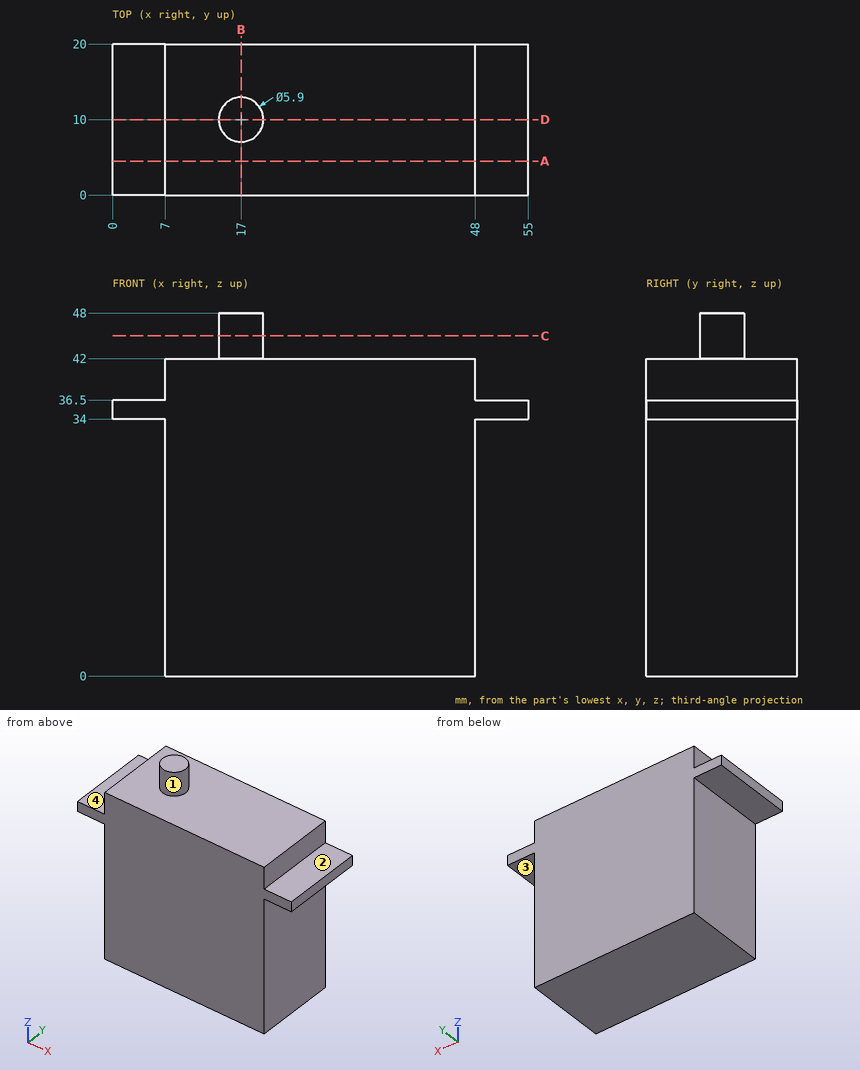
Here's the drawing with two shaded views (mm, measured from the low corner). I have some questions. A direction names the side the tool comes from. Give positions to 0.01 mm unless a question says otherwise; leave off trailing zeros. Order: outer loops, then holes, each group sorted by start corner. A loop starts at its lowest first (then second) coordinate and runs counter-clockwise, first axis right, second up. Notation, with made-up numbers: (72, 55) -> (79, 55) arc R35 cw to (79, 93) -> close; hole circle Ø6 at (89, -15.75). An arc over 180 degrees is marked (long way). One line per item, written item: value. Start each with the question number.
1. Will these pins go through, and if not, where does the flat tip stop? pin 1 Ø1 at (x, z) = (47, 21) entering from -Y; pin 2 Ø1.5 at (y, z) = (8, 29.5) entering from +X; pin 3 Ø3.5 at (x, y) = (4.5, 8.5) entering from +Z; pin 4 Ø3.5 at (x, y) = (53, 14) entering from -Z.
2. Imagine slicing it at A-A, the plane y = 4.5. List the corners of the cut face in (x, z) for me.
3. Imagine slicing it at D-D, the plane y = 10. List the corners of the cut face in (x, z) for me.
4. Imagine slicing it at B-B, the plane x = 17. List the corners of the cut face in (y, z) for me, plus the area to 3 significant figures.
5. Imagine slicing it at C-C, the plane z = 45. List the corners of the cut face in (x, y) for me, plus the area to 3 significant figures.
6. For the marked faces 1, 2, 3 and 4, which set-ups out of +Z, -Z, +X, -X, +Y, -Y let a thin tool reach every point of the face, with its end or its side?
7. I need wall thicknesses on probe 1 along Z at (x, y) = (9.5, 9); probe 2 along X at (y, z) = (1.75, 23); probe 3 along Z at (x, y) = (5.5, 7). Which ranges of each line are inside material? Lowest first, please. Write a range as from..to.
Values follow:
1. pin 1: stops at y = 0
1. pin 2: stops at x = 48
1. pin 3: stops at z = 36.5
1. pin 4: stops at z = 34
2. outline: (0, 34) -> (7, 34) -> (7, 0) -> (48, 0) -> (48, 34) -> (55, 34) -> (55, 36.5) -> (48, 36.5) -> (48, 42) -> (7, 42) -> (7, 36.5) -> (0, 36.5) -> close
3. outline: (0, 34) -> (7, 34) -> (7, 0) -> (48, 0) -> (48, 34) -> (55, 34) -> (55, 36.5) -> (48, 36.5) -> (48, 42) -> (19.95, 42) -> (19.95, 48) -> (14.05, 48) -> (14.05, 42) -> (7, 42) -> (7, 36.5) -> (0, 36.5) -> close
4. outline: (0, 0) -> (20, 0) -> (20, 42) -> (12.95, 42) -> (12.95, 48) -> (7.05, 48) -> (7.05, 42) -> (0, 42) -> close
4. area: 875 mm2
5. outline: circle Ø5.9 at (17, 10)
5. area: 27.3 mm2
6. face 1: +Z
6. face 2: +Z, +X, +Y, -Y
6. face 3: -Z, +X, +Y, -Y
6. face 4: +Z, -X, +Y, -Y
7. probe 1: z = 0..42
7. probe 2: x = 7..48
7. probe 3: z = 34..36.5
